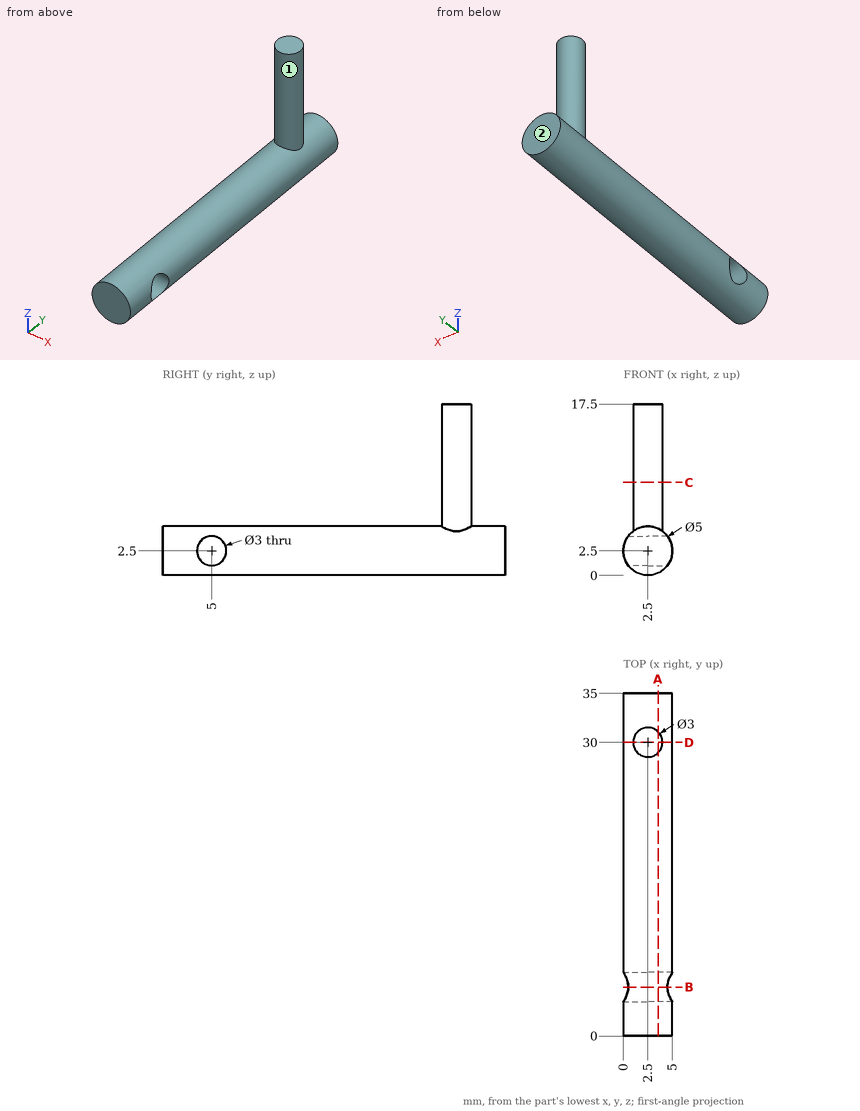
Verification items for this drawing (mm, ordinates from the low corner). A direction names the side the tool comes from. Coordinates: 2 decimals unless noted, no trailing zeros. Write each loop counter-clockwise with the first axis right and the second up, starting at its lowest first coordinate (ties: lowest second). Pieces come first, ordered by that corner, then holes. Notation, with made-up numbers: M 46,-8 L 72,-8 A18 ccw 72,16 Z; hole C 80.25,63 d6. An arc over 180 degrees is marked long. Use one line per item in the form item = value. Start each with the question number.
1) Set-up check for the marked faces 1 and 2: record each of +Z, -Z, +X, -X, +Y, -Y from which the full face is reachable in a straight line by a thin tool's end or side.
2) Section check C-C on z = 9.5. Enter the section's corners in (x, y).
3) Section check A-A on x = 3.55. Enter the section's corners in (y, z).
4) Thickness scan on probe 1 along Y at (x, z) = (4.4, 2.5); probe 2 along Y at (x, z) = (1.4, 3.5); probe 3 along Y at (x, z) = (2.45, 14). Record the ranges inside material, lowest first. Write a range as from..to.
5) Go/stop test with flat-tipped pins: pin 1 Ø6 at (y, z) = (13.5, 2) entering from +X; pin 2 Ø8 at (y, z) = (19.5, 8.5) entering from -X; pin 3 Ø2 at (x, z) = (3, 9.5) entering from -Y. Record where each tip stops, or that it passes through.
6) Section check B-B on y = 5. Enter the section's corners in (x, z).
7) Section check D-D on y = 30. Enter the section's corners in (x, z).
Responses:
q1.face_1 = +Z
q1.face_2 = +Z, -Z, +X, -X, +Y
q2.outline = C 2.5,30 d3
q3.outline = M 0,0.23 L 35,0.23 L 35,4.77 L 31.07,4.77 L 31.07,17.5 L 28.93,17.5 L 28.93,4.77 L 0,4.77 Z; hole C 5,2.5 d3
q4.probe_1 = 0..3.5, 6.5..35
q4.probe_2 = 0..3.88, 6.12..35
q4.probe_3 = 28.5..31.5
q5.pin_1 = 5
q5.pin_2 = 1
q5.pin_3 = 28.5
q6.outline = M 0.5,1 A2.5 ccw 4.5,1 Z; M 0.5,4 L 4.5,4 A2.5 ccw Z
q7.outline = M 1,4.5 A2.5 ccw long 4,4.5 L 4,17.5 L 1,17.5 Z
